Geometry check sheet. Reference: the model listing, model coordinates, mm. A direction names the side the tool comes from. Give positions to 0.01 mm unless a question says otherwise; leave off trailing zeros. Loops run counter-clockwise (first coordinate to the right, second up) from the corner with the lowest first, then second, coordinate; pieces in that order, holes last. Notation, with made-up numbers: (28.5, -10) -> (41.5, -10) arc R8 ccw to (41.5, 3) -> close; hole circle Ø10 at (19.25, 34). An arc over 180 degrees is marked (long way). One line per question, with ' | ' between items.
from build123d import *

# Parameters (mm, degrees)
BOSS_EXTRUDE1_DEPTH       = 15.875
F_6_32_TAPPED_HOLE1_D     = 2.7051
F_6_32_TAPPED_HOLE1_DEPTH = 5.08
F_6_32_TAPPED_HOLE1_TIP   = 0.81269403
F_6_32_TAPPED_HOLE2_D     = 2.7051
F_6_32_TAPPED_HOLE2_DEPTH = 5.08
F_6_32_TAPPED_HOLE2_TIP   = 0.81269403


with BuildPart() as part:
    # Sketch2 → Boss-Extrude1 (new body)
    with BuildSketch(Plane(origin=(0, 0, 0), x_dir=(1, 0, 0), z_dir=(0, 1, 0))):
        Polygon((4.582717762, 0), (2.291358881, 3.96875), (-2.291358881, 3.96875), (-4.582717762, 0), (-2.291358881, -3.96875), (2.291358881, -3.96875), align=None)
    extrude(amount=BOSS_EXTRUDE1_DEPTH)

    # #6-32 Tapped Hole1
    with Locations(Plane(origin=(0, 0, 0), x_dir=(-1, 0, 0), z_dir=(0, -1, 0))):
        with Locations((0, 0)):
            Hole(F_6_32_TAPPED_HOLE1_D / 2, depth=F_6_32_TAPPED_HOLE1_DEPTH)
            with Locations((0, 0, -(F_6_32_TAPPED_HOLE1_DEPTH + F_6_32_TAPPED_HOLE1_TIP / 2))):  # 118° drill point
                Cone(0, F_6_32_TAPPED_HOLE1_D / 2, F_6_32_TAPPED_HOLE1_TIP, mode=Mode.SUBTRACT)

    # #6-32 Tapped Hole2
    with Locations(Plane(origin=(0, 15.875, 0), x_dir=(1, 0, 0), z_dir=(0, 1, 0))):
        with Locations((0, 0)):
            Hole(F_6_32_TAPPED_HOLE2_D / 2, depth=F_6_32_TAPPED_HOLE2_DEPTH)
            with Locations((0, 0, -(F_6_32_TAPPED_HOLE2_DEPTH + F_6_32_TAPPED_HOLE2_TIP / 2))):  # 118° drill point
                Cone(0, F_6_32_TAPPED_HOLE2_D / 2, F_6_32_TAPPED_HOLE2_TIP, mode=Mode.SUBTRACT)


solid = part.part
Item 1: Depth check by flat-ended pin: pin 1 Ø2.5 at (x, z) = (0, 0) entering from +Y; pin 2 Ø2 at (y, z) = (10.5, -1.5) entering from -X. Enter the tip coordinate at first touch or a pass-through.
Result:
pin 1: y = 10.73 | pin 2: x = -4.29
Item 2: Sectioned sample at C-C (z = -3.5). Record the cut outline in (x, y) (3 decimals).
Result:
outline: (-2.562, 0) -> (2.562, 0) -> (2.562, 15.875) -> (-2.562, 15.875) -> close
Item 3: Set-up check for faces 1 (the face through (3.45, 7.83, -1.96)), 2 (the face through (-1.29, 13.3, -0.41)), 3 (the face through (1.29, 2.58, -0.41)): record each of +Z, -Z, +X, -X, +Y, -Y from which the full face is reachable in a straight line by a thin tool's end or side.
Result:
face 1: -Z, +X, +Y, -Y | face 2: +Y | face 3: -Y
Item 4: Release check for a two-part mould opening along X. For faces 4 (the face through (-3.45, 7.83, 1.96)), 5 (the face through (0.05, 5.75, 0.23)), 6 (the face through (0, 0, 2)) record: pulls with the +X half, pulls with the -X half, needs draft (parallel to the pull), parting line crosses it, or undercut.
Result:
face 4: pulls with the -X half | face 5: undercut | face 6: needs draft
Item 5: Scan lines: probe 1 along Z at (x, y) = (0, 13.85); probe 2 along Z at (x, y) = (0.75, 14.75); probe 3 along Z at (x, y) = (-3.75, 9.5). Record each from-to range of solid material in increasing order.
Result:
probe 1: -3.97 to -1.35, 1.35 to 3.97 | probe 2: -3.97 to -1.13, 1.13 to 3.97 | probe 3: -1.44 to 1.44
Item 6: Sectioned sample at B-B (y = 7.25). Record the cut outline in (x, z), plus the area to 3 significant figures.
Result:
outline: (-4.58, 0) -> (-2.29, -3.97) -> (2.29, -3.97) -> (4.58, 0) -> (2.29, 3.97) -> (-2.29, 3.97) -> close | area: 54.6 mm2
Item 7: Sectioned sample at D-D (z = -2.25). Record the cut outline in (x, y) (3 decimals).
Result:
outline: (-3.284, 0) -> (3.284, 0) -> (3.284, 15.875) -> (-3.284, 15.875) -> close
Item 8: Sectioned sample at A-A (y = 13). Record the cut outline in (x, z).
Result:
outline: (-4.58, 0) -> (-2.29, -3.97) -> (2.29, -3.97) -> (4.58, 0) -> (2.29, 3.97) -> (-2.29, 3.97) -> close; hole circle Ø2.71 at (0, 0)
